Check sheet for the modelled part. Datum: model origin and axes. Units: mm. Face numbers are marked on the shaded views. A direction names the side the tool comes from. Round coordinates to 2 decimals unless told otherwise and drop trailing zeros. Order: outer loops, then holes, each group sorted by start corner. A loop starts at its lowest first (then second) coordinate and runs counter-clockwise, first axis right, second up.
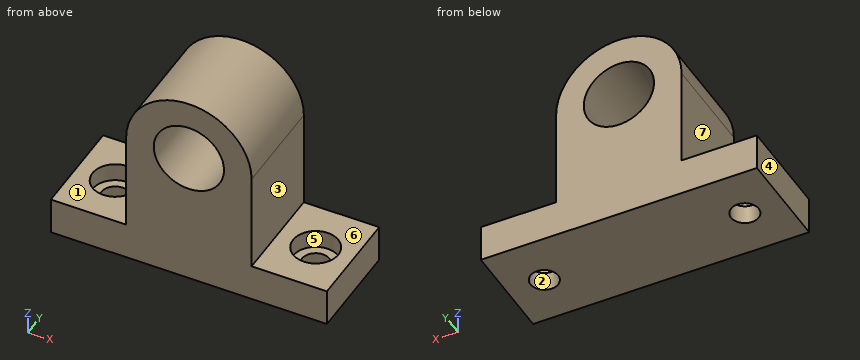
from build123d import *

# Parameters (mm, degrees)
F0_R     = 14
F1_DEPTH = 40
F2_R     = 9
F2_R_2   = 5.5
F3_DEPTH = 7.3
F4_DEPTH = 15


with BuildPart() as f1:
    # F0 (on Front) → F1 (new body)
    with BuildSketch(Plane.XZ):
        with BuildLine():
            Line((-55, -27.2687692195), (0, -27.2687692195))
            Line((0, -27.2687692195), (55, -27.2687692195))
            Line((55, -27.2687692195), (55, -12.2687692195))
            Line((55, -12.2687692195), (25, -12.2687692195))
            Line((25, -12.2687692195), (25, 27.7312307805))
            ThreePointArc((25, 27.7312307805), (0, 52.7312307805), (-25, 27.7312307805))
            Line((-25, 27.7312307805), (-25, -12.2687692195))
            Line((-25, -12.2687692195), (-55, -12.2687692195))
            Line((-55, -12.2687692195), (-55, -27.2687692195))
        make_face()
        with Locations((0, 27.7312307805)):
            Circle(F0_R, mode=Mode.SUBTRACT)
    extrude(amount=F1_DEPTH)

    # F2 (on face) → F3 (cut)
    with BuildSketch(Plane.XY.offset(-12.2687692195)):
        with Locations((40.221106261, -20.1945845038)):
            Circle(F2_R)
        with Locations((40.221106261, -20.1945845038)):
            Circle(F2_R_2, mode=Mode.SUBTRACT)
        with Locations((-39.6916903555, -20.1945845038)):
            Circle(F2_R)
        with Locations((-39.6916903555, -20.1945845038)):
            Circle(F2_R_2, mode=Mode.SUBTRACT)
    extrude(amount=-F3_DEPTH, mode=Mode.SUBTRACT)

    # F4 (cut): faces of the model
    f4_faces = [f1.faces().sort_by_distance(p)[0] for p in [
        (-39.6916903555, -20.1945845038, -12.2687692195),
        (40.221106261, -20.1945845038, -12.2687692195),
    ]]
    extrude(f4_faces, amount=-F4_DEPTH, mode=Mode.SUBTRACT)


solid = f1.part
1) Sectioned sample at A-A on x = 0. Record the cut outline in (y, z).
2) Sectioned sample at B-B on y = -31.5. Record the cut outline in (x, z).
3) Sectioned sample at D-D on z = -1.5. Record the cut outline in (x, y), and give its area (3 significant figures).
4) Draft check along X on the marked faces 1, 2, 3 and 4. Enter one of: pulls with the +X half, pulls with the -X half, needs draft (parallel to the pull), parting line crosses it, or undercut.
5) Sectioned sample at C-C on z = -22. Record the cut outline in (x, y).
6) Scan lines: line 1 (Z direction, x = 0, y = -12); line 2 (Z direction, x = -36, y = -5); line 3 (X direction, y = -24, z = 31). Record each from-to range of solid material in increasing order.
7) Gauge pin test, flat ends, axial feed: pin 1 (1 mm diameter, centred on y = -34, z = 42.5, fed in from +X); pin 2 (9 mm diameter, centred on x = -41, y = -11, fed in from +Z); pin 3 (12.5 mm diameter, centred on x = -39.69, y = -20.19, fed in from +Z); pin 4 (6.5 mm diameter, centred on x = 40.22, y = -20.19, fed in from +Z). Record the tip position at first contact, or that the pin passes through.
8) Set-up check for the marked faces 5, 6 and 7: record each of +Z, -Z, +X, -X, +Y, -Y from which the full face is reachable in a straight line by a thin tool's end or side.
Values found:
1. outline: (-40, -27.27) - (0, -27.27) - (0, 13.73) - (-40, 13.73) - close; (-40, 41.73) - (0, 41.73) - (0, 52.73) - (-40, 52.73) - close
2. outline: (-55, -27.27) - (55, -27.27) - (55, -12.27) - (25, -12.27) - (25, 27.73) arc R25 ccw to (-25, 27.73) - (-25, -12.27) - (-55, -12.27) - close; hole circle Ø28 at (0, 27.73)
3. outline: (-25, -40) - (25, -40) - (25, 0) - (-25, 0) - close
3. area: 2,000 mm2
4. face 1: needs draft
4. face 2: undercut
4. face 3: pulls with the +X half
4. face 4: pulls with the -X half
5. outline: (-55, -40) - (55, -40) - (55, 0) - (-55, 0) - close; hole circle Ø11 at (-39.69, -20.19); hole circle Ø11 at (40.22, -20.19)
6. line 1: z = -27.27 to 13.73, 41.73 to 52.73
6. line 2: z = -27.27 to -12.27
6. line 3: x = -24.79 to -13.61, 13.61 to 24.79
7. pin 1: stops at x = 20.53
7. pin 2: stops at z = -12.27
7. pin 3: stops at z = -19.57
7. pin 4: passes through
8. face 5: +Z
8. face 6: +Z, +X, +Y, -Y
8. face 7: +Z, -X, +Y, -Y
